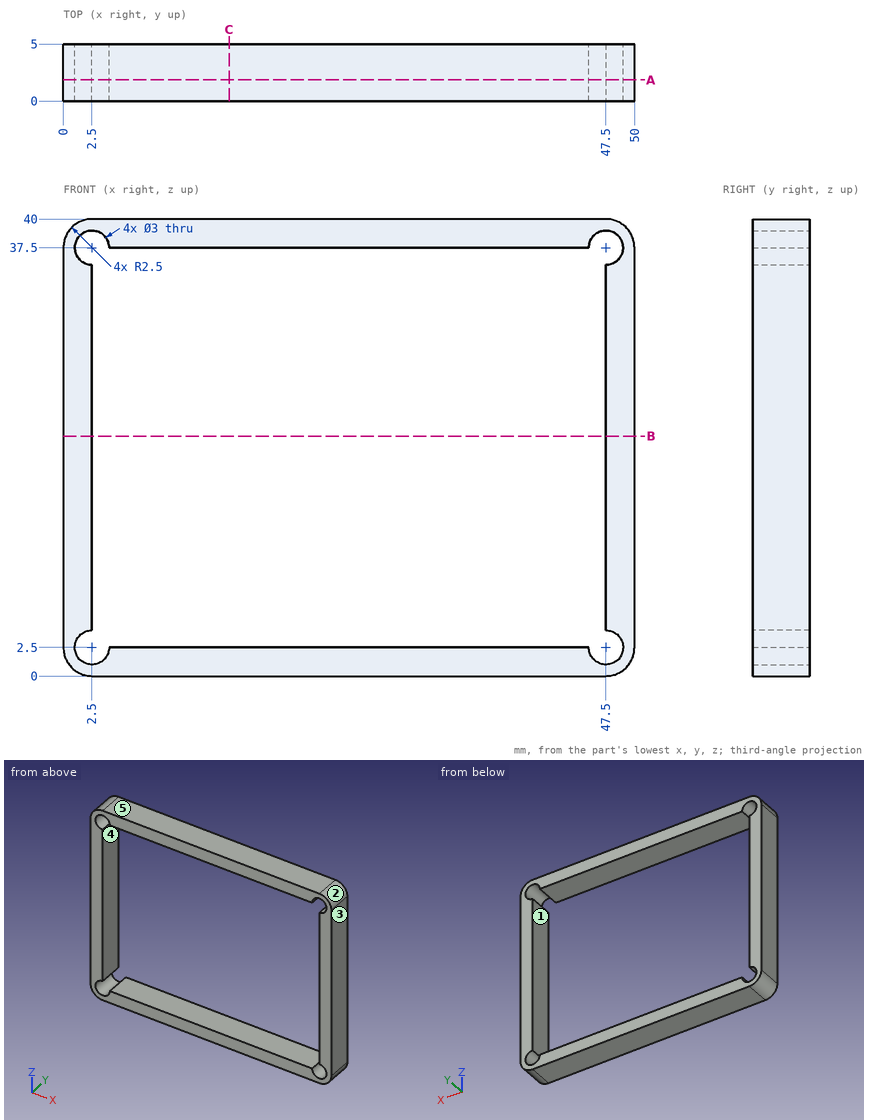
The figure shows three views and two pictorial views of one solid part (mm, origin at its lowest corner). Answer the questions. A direction names the side the tool comes from. Coordinates: 2 decimals unless noted, no trailing zeros. Loops run counter-clockwise (first coordinate to the right, second up) from the corner with the lowest first, then second, coordinate; pieces in that order, holes last. Notation, with made-up numbers: (83.5, 68.25) - (96.5, 68.25) arc R32 cw to (96.5, 105.25) - close; hole circle Ø3 at (22.5, 86.25). An arc over 180 degrees is marked (long way). Answer in a Markdown table with one row per item.
Q1. Find section B-B on z = 21. Write down the section's boundary in (x, y).
Here are the results:
| item | result |
|---|---|
| outline | (0, 0) - (2.5, 0) - (2.5, 5) - (0, 5) - close; (47.5, 0) - (50, 0) - (50, 5) - (47.5, 5) - close |
Q2. Find section A-A on y = 1.85. Write down the section's boundary in (x, z), plus the area to 3 significant figures.
Here are the results:
| item | result |
|---|---|
| outline | (0, 2.5) arc R2.5 ccw to (2.5, 0) - (47.5, 0) arc R2.5 ccw to (50, 2.5) - (50, 37.5) arc R2.5 ccw to (47.5, 40) - (2.5, 40) arc R2.5 ccw to (0, 37.5) - close; hole (2.5, 4) arc R1.5 ccw (long way) to (4, 2.5) - (46, 2.5) arc R1.5 ccw (long way) to (47.5, 4) - (47.5, 36) arc R1.5 ccw (long way) to (46, 37.5) - (4, 37.5) arc R1.5 ccw (long way) to (2.5, 36) - close |
| area | 398 mm^2 |
Q3. Straight lines are drawn through the part: line 1 along X through (y, z) = (1.6, 30.5); line 2 along Z through (x, y) = (35.5, 3.9); line 3 along X through (y, z) = (3.7, 38). For each, find the intervals that lie inside material, in ascending order. Write a range as [from, to].
Here are the results:
| item | result |
|---|---|
| line 1 | x = [0, 2.5], [47.5, 50] |
| line 2 | z = [0, 2.5], [37.5, 40] |
| line 3 | x = [0.05, 1.09], [3.91, 46.09], [48.91, 49.95] |
Q4. The mould has two halves that part along Z. Classify the marked faces 1, 2 and 3: pulls with the +Z half, pulls with the -Z half, needs draft (parallel to the pull), parting line crosses it, or undercut.
Here are the results:
| item | result |
|---|---|
| face 1 | undercut |
| face 2 | pulls with the +Z half |
| face 3 | needs draft |
Q5. Find section C-C on x = 14.5. Write down the section's boundary in (y, z), plus the area to 3 significant figures.
Here are the results:
| item | result |
|---|---|
| outline | (0, 0) - (5, 0) - (5, 2.5) - (0, 2.5) - close; (0, 37.5) - (5, 37.5) - (5, 40) - (0, 40) - close |
| area | 25.0 mm^2 |
Q6. For the marked faces 4 and 5, determine the directions among +Z, -Z, +X, -X, +Y, -Y from which every point of the face is accessible in a straight line to the end or side of a thin tool.
Here are the results:
| item | result |
|---|---|
| face 4 | +Y, -Y |
| face 5 | +Z, +X, -X, +Y, -Y |
